Read the model definition and answer for the solid it produces. Units are mm, in the model's axes. Coordinates: 2 decimals unless noted, no trailing zeros. Loops run counter-clockwise (first coordinate to the right, second up) from the corner with the lowest first, then second, coordinate; pieces in that order, holes last. Notation, with made-up numbers: (60, 23.5) -> (115, 23.5) arc R9 ccw to (115, 39.5) -> close; hole circle Ø11 at (88.5, 13). An arc over 180 degrees is marked (long way). Answer as a JSON object with one key per item and string values. Group by question number.
Q1. Straight lines are drawn through the part: line 1 along X through (y, z) = (-143.9, -2.5); line 2 along Y through (x, z) = (180, -0.2); line 3 along Y through (x, z) = (204, -3.35). For each, find the intervals that lie inside material, in ascending order. Write a range as [from, to].
Q2. The part is cut by section C-C on y = -60.5. Write down the section's boundary in (x, z), and give its area (4 significant figures).
Q3. Each of these flat-tipped pins is pushed along its axis until it touches: P1, Ø5, axis at x = 203.32, y = -114.1, coming from the -Z side; P2, Ø3.5, axis at x = 169.32, y = -60.5, coming from the +Z side. Where does it stop, or does it pass through?
Q4. The part is cut by section B-B on y = -114.1. Write down the section's boundary in (x, z), and give its area (4 significant figures).
Q5. The part is cut by section A-A on z = -2.85. State how many separate pieces and enclosed holes the cut face has, and give its area (3 significant figures).
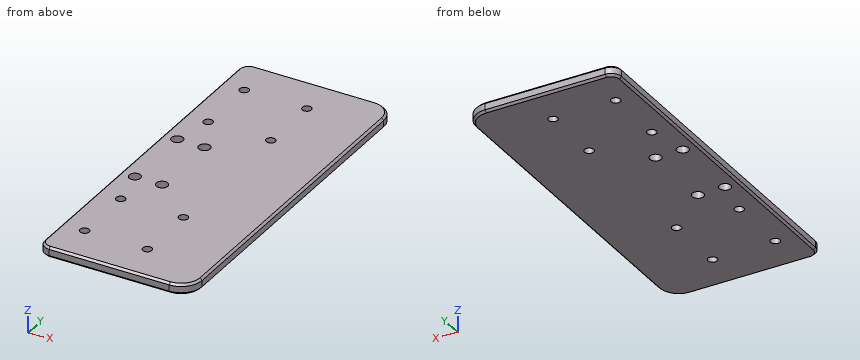
from build123d import *

# Parameters (mm, degrees)
EXTRUDE_1_DEPTH     = 5
SKETCH_4_R          = 2.2
SKETCH_4_R_2        = 2.75
CUT_EXTRUDE_1_DEPTH = 5
CHAMFER_2_SIZE      = 1


with BuildPart() as part:
    # 草图1 → 凸台-拉伸1 (new body)
    with BuildSketch(Plane.XY):
        with BuildLine():
            Line((234.824487649, -3.000003036), (234.824487649, -152.999988316))
            ThreePointArc((234.824487649, -152.999988316), (231.895556179, -160.071055409), (224.824489681, -162.999988316))
            Line((224.824489681, -162.999988316), (167.324488665, -163))
            ThreePointArc((167.324488665, -163), (163.788954102, -161.535534265), (162.324487649, -158))
            Line((162.324487649, -158), (162.324487649, 2))
            ThreePointArc((162.324487649, 2), (163.788953837, 5.535533999), (167.324487913, 7))
            Line((167.324487913, 7), (224.824488177, 6.999996964))
            ThreePointArc((224.824488177, 6.999996964), (231.895555648, 4.071064589), (234.824487649, -3.000003036))
        make_face()
    extrude(amount=-EXTRUDE_1_DEPTH)

    # 草图4 → 切除-拉伸1 (cut)
    with BuildSketch(Plane.XY):
        with Locations((203.324487649, -12.1)):
            Circle(SKETCH_4_R)
        with Locations((173.324487649, -12.1)):
            Circle(SKETCH_4_R)
        with Locations((173.324487649, -41.9)):
            Circle(SKETCH_4_R)
        with Locations((203.324487649, -41.9)):
            Circle(SKETCH_4_R)
        with Locations((173.324487649, -143.9)):
            Circle(SKETCH_4_R)
        with Locations((203.324487649, -143.9)):
            Circle(SKETCH_4_R)
        with Locations((173.324487649, -114.1)):
            Circle(SKETCH_4_R)
        with Locations((203.324487649, -114.1)):
            Circle(SKETCH_4_R)
        with Locations((169.324487649, -60.5)):
            Circle(SKETCH_4_R_2)
        with Locations((169.324487649, -95.5)):
            Circle(SKETCH_4_R_2)
        with Locations((182.324487649, -60.5)):
            Circle(SKETCH_4_R_2)
        with Locations((182.324487649, -95.5)):
            Circle(SKETCH_4_R_2)
    extrude(amount=-CUT_EXTRUDE_1_DEPTH, mode=Mode.SUBTRACT)

    # 倒角2
    chamfer_2_edges = [part.edges().sort_by_distance(p)[0] for p in [
        (196.074489173, -162.999994158, 0),
        (163.788954102, -161.535534265, 0),
        (231.895555648, 4.071064589, -5),
        (162.324487649, -78, 0),
        (163.788953837, 5.535533999, 0),
        (196.074488045, 6.999998482, 0),
        (231.895555648, 4.071064589, 0),
        (234.824487649, -77.999995676, 0),
        (196.074488045, 6.999998482, -5),
        (163.788953837, 5.535533999, -5),
        (162.324487649, -78, -5),
        (163.788954102, -161.535534265, -5),
        (196.074489173, -162.999994158, -5),
        (231.895556179, -160.071055409, -5),
        (234.824487649, -77.999995676, -5),
        (231.895556179, -160.071055409, 0),
    ]]
    chamfer(chamfer_2_edges, length=CHAMFER_2_SIZE)


solid = part.part
Final values:
{
 "1": {"line 1": "x = [162.32, 171.12], [175.52, 201.12], [205.52, 234.82]", "line 2": "y = [-162.2, -96.97], [-94.03, -61.97], [-59.03, 6.2]", "line 3": "y = [-163, -145.99], [-141.81, -116.19], [-112.01, -43.99], [-39.81, -14.19], [-10.01, 7]"},
 "2": {"outline": "(162.32, -4) -> (163.32, -5) -> (166.57, -5) -> (166.57, 0) -> (163.32, 0) -> (162.32, -1) -> close; (172.07, -5) -> (179.57, -5) -> (179.57, 0) -> (172.07, 0) -> close; (185.07, -5) -> (233.82, -5) -> (234.82, -4) -> (234.82, -1) -> (233.82, 0) -> (185.07, 0) -> close", "area": "305.5 mm2"},
 "3": {"P1": "stops at z = -5", "P2": "passes through"},
 "4": {"outline": "(162.32, -4) -> (163.32, -5) -> (171.12, -5) -> (171.12, 0) -> (163.32, 0) -> (162.32, -1) -> close; (175.52, -5) -> (201.12, -5) -> (201.12, 0) -> (175.52, 0) -> close; (205.52, -5) -> (233.82, -5) -> (234.82, -4) -> (234.82, -1) -> (233.82, 0) -> (205.52, 0) -> close", "area": "316.5 mm2"},
 "5": {"separate pieces": "1", "enclosed holes": "12", "area": "12,100 mm2"}
}
